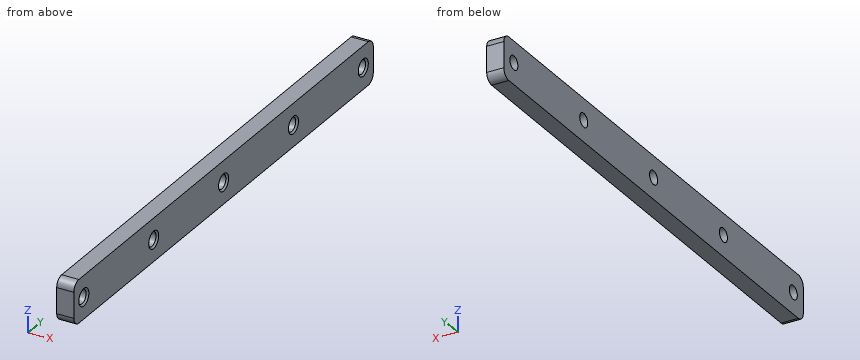
```python
from build123d import *

# Parameters (mm, degrees)
F0_W           = 10
F0_H           = 300
F1_DEPTH       = 25
F3_D           = 8
F3_CSINK_D     = 10
F3_CSINK_ANGLE = 90
F4_R           = 5


with BuildPart() as f1:
    # F0 (on Top) → F1 (new body)
    with BuildSketch(Plane.XY):
        with Locations((-5, 150)):
            Rectangle(F0_W, F0_H)
    extrude(amount=F1_DEPTH)

    # F3 (through all)
    with Locations(Plane.YZ):
        with Locations((10, 12.5), (80, 12.5), (150, 12.5), (220, 12.5), (290, 12.5)):
            CounterSinkHole(F3_D / 2, F3_CSINK_D / 2, counter_sink_angle=F3_CSINK_ANGLE)

    # F4
    f4_edges = [f1.edges().sort_by_distance(p)[0] for p in [
        (-5, 0, 0),
        (-5, 300, 0),
        (-5, 0, 25),
        (-5, 300, 25),
    ]]
    fillet(f4_edges, radius=F4_R)


solid = f1.part
```
Verification items for the finished model (mm, model axes). Round coordinates to 2 decimals unless told otherwise and drop trailing zeros. Write each loop counter-clockwise with the first axis right and the second up, starting at its lowest first coordinate (ties: lowest second). Pieces come first, ordered by that corner, then holes. Notation, with made-up numbers: (-23.75, 57.25) - (-18.75, 57.25) arc R18 cw to (-18.75, 73.25) - close; hole circle Ø2 at (55.25, 45). An arc over 180 degrees is marked (long way). Answer as a JSON object with one key per item and string values. Group by question number.
Q1. Thickness scan on line 1 (Y direction, x = -4, z = 12.5); line 2 (Z direction, x = -6, y = 220); line 3 (Y direction, x = -4, z = 14). Record the ranges inside material, lowest first.
Q2. Section check A-A, the plane y = 290. Enter the section's corners in (x, z), plus the area to 3 significant figures.
Q3. Section check C-C, the plane z = 12.5. Give the number of separate pieces and of enclosed holes in the cut face, plus the area to 4 significant figures.
Q4. Go/stop test with flat-tipped pins: pin 1 Ø6.5 at (y, z) = (150, 12.5) entering from +X; pin 2 Ø9 at (y, z) = (220, 12.5) entering from -X; pin 3 Ø3 at (x, z) = (-6, 22) entering from +Y. Record where each tip stops, or that it passes through.
Q5. Section check B-B, the plane x = -5. Enter the section's corners in (y, z).
Found:
{
 "1": {"line 1": "y = 0 to 6, 14 to 76, 84 to 146, 154 to 216, 224 to 286, 294 to 300", "line 2": "z = 0 to 8.5, 16.5 to 25", "line 3": "y = 0 to 6.29, 13.71 to 76.29, 83.71 to 146.29, 153.71 to 216.29, 223.71 to 286.29, 293.71 to 300"},
 "2": {"outline": "(-10, 0) - (0, 0) - (0, 7.5) - (-1, 8.5) - (-10, 8.5) - close; (-10, 16.5) - (-1, 16.5) - (0, 17.5) - (0, 25) - (-10, 25) - close", "area": "169 mm^2"},
 "3": {"separate pieces": "6", "enclosed holes": "0", "area": "2,595 mm^2"},
 "4": {"pin 1": "passes through", "pin 2": "stops at x = -10", "pin 3": "stops at y = 299.97"},
 "5": {"outline": "(0, 5) arc R5 ccw to (5, 0) - (295, 0) arc R5 ccw to (300, 5) - (300, 20) arc R5 ccw to (295, 25) - (5, 25) arc R5 ccw to (0, 20) - close; hole circle Ø8 at (10, 12.5); hole circle Ø8 at (80, 12.5); hole circle Ø8 at (150, 12.5); hole circle Ø8 at (220, 12.5); hole circle Ø8 at (290, 12.5)"}
}
